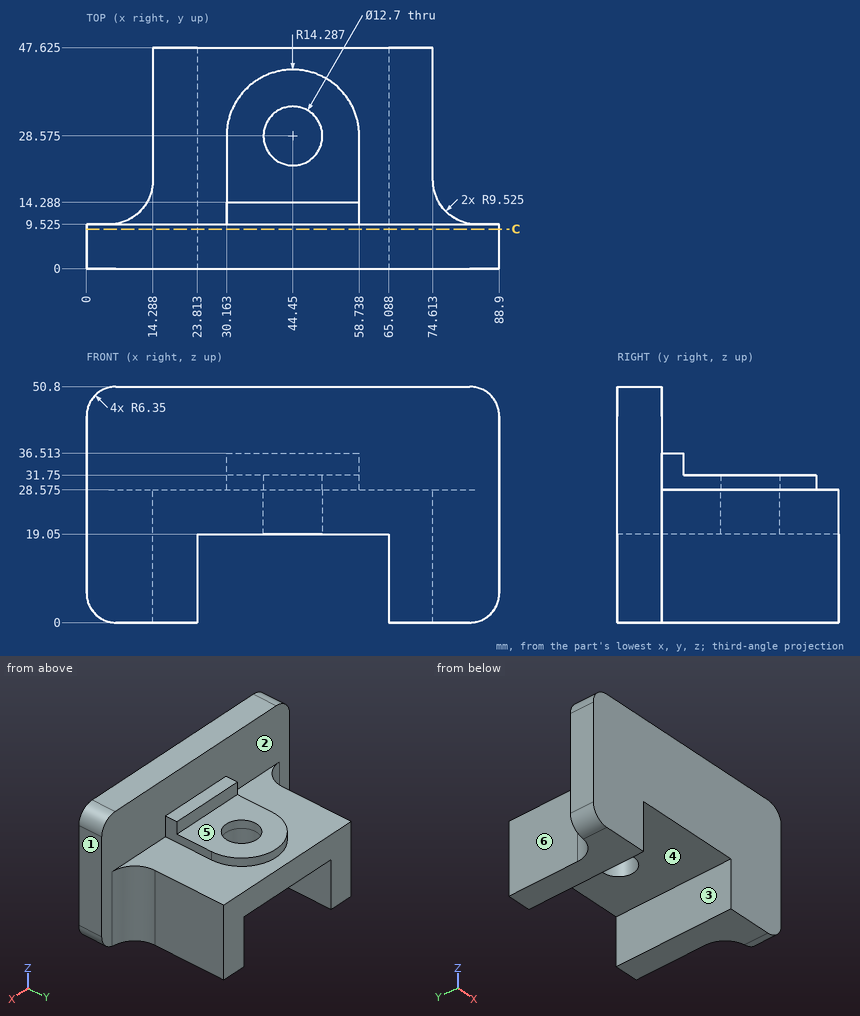
Input: dimensioned drawing with shaded views. Units: mm. Origin: part minimum x, y, z. A direction names the side the tool comes from. Coordinates: 2 decimals unless noted, no trailing zeros. Order: outer loops, then holes, each group sorted by start corner. A loop starts at its lowest first (then second) coordinate and runs counter-clockwise, first axis right, second up.
Item 1: Draft query along X for the marked faces 1, 2 and 3. Return one class per face: released by +X, released by -X, zero draft, split by the parting line, or undercut.
Answer:
face 1: released by +X
face 2: zero draft
face 3: undercut
Item 2: Section query C-C (y = 8.5). Output: boundary loops of the cut face in (x, z).
Answer:
outline: (0, 6.35) arc R6.35 ccw to (6.35, 0) - (23.81, 0) - (23.81, 19.05) - (65.09, 19.05) - (65.09, 0) - (82.55, 0) arc R6.35 ccw to (88.9, 6.35) - (88.9, 44.45) arc R6.35 ccw to (82.55, 50.8) - (6.35, 50.8) arc R6.35 ccw to (0, 44.45) - close
Item 3: Contact query for flat-ended pins moving along their axis: P1, Ø5, axis at x = 55.5, y = 37, coming from the -Z side; P2, Ø5, axis at y = 26.5, z = 5.5, coming from the -X side; P3, Ø2.5, axis at y = 16.5, z = 32.5, coming from the -X side; P4, Ø11.5, axis at x = 44.45, y = 28.575, coming from the -Z side. Output: stop coordinate, or through.
Answer:
P1: stops at z = 19.05
P2: stops at x = 14.29
P3: stops at x = 30.16
P4: passes through
Item 4: Material intervals for line 1 along Y through (x, z) = (44.45, 29.35) (1 decimal); line 2 along Y through (x, z) = (44.45, 24) (1 decimal); line 3 along Y through (x, z) = (25.5, 39) (1 decimal), sorted ascending.
Answer:
line 1: y = 0 to 22.2, 34.9 to 42.9
line 2: y = 0 to 22.2, 34.9 to 47.6
line 3: y = 0 to 9.5
Item 5: Access query for the marked faces 4, 5 and 6. Directions: +Z, -Z, +X, -X, +Y, -Y. A direction counts if a zero-diameter tool reaches every point of the face in a straight line with its end or side. Return the directions, or none.
Answer:
face 4: -Z, +Y, -Y
face 5: +Z, +X, -X, +Y
face 6: +Z, -Z, -X, +Y
